CAD build for the part. Positions are in the model's coordinates, mm. A direction names the side the tool comes from. Give positions to 0.01 mm unless a question says otherwise; leave off trailing zeros. Order: outer loops, then holes, each group sorted by start corner. A loop starts at its lowest first (then second) coordinate and runs counter-clockwise, first axis right, second up. Notation, with made-up numbers: (58, 52) -> (77, 52) arc R27 cw to (77, 83) -> close; hole circle Ø5 at (20.25, -18). An arc over 180 degrees is marked (long way). Answer as CSV lines item,"result".
Autodesk Inventor part; units mm, degrees
ref_plane "YZ Plane" through (0, 0, 0) normal (1, 0, 0) x (0, 1, 0)
ref_plane "XZ Plane" through (0, 0, 0) normal (0, 1, 0) x (-1, 0, 0)
ref_plane "XY Plane" through (0, 0, 0) normal (0, 0, 1) x (1, 0, 0)
sketch "Эскиз4" plane through (0, 0, 0) normal (0, 1, 0) x (-1, 0, 0)
  line L0 (20.7, 60) -> (23.2, 6)
  line L1 (25, 6) -> (22.5, 60)
  line L2 (0, -13.2) -> (0, 79.2) construction
  line L3 (25, 6) -> (23.2, 6) construction
  line L4 (23.2, 6) -> (23.2, 0)
  line L5 (23.2, 0) -> (25, 0)
  line L6 (25, 0) -> (25, 6)
  line L7 (22.5, 60) -> (20.7, 60) construction
  line L8 (20.7, 60) -> (20.7, 66)
  line L9 (20.7, 66) -> (22.5, 66)
  line L10 (22.5, 66) -> (22.5, 60)
  line L11 (25.86, 0) -> (19.84, 0) construction
  dimension "d11" = 25
  dimension "d13" = 22.5
  dimension "d16" = 6
  dimension "d17" = 1.8
  dimension "d18" = 66
revolve "Вращение1" add sketch "Эскиз4" angle 360 about axis through (0, 0, -10) along (0, 0, 1)
properties part number "Конусный барабан катушки"
1) Wall check: line 1 along Y through (x, z) = (0, 61.9); line 2 along Y through (x, z) = (0, 2). Give the ranges that are in metal, low to high. Write a range as [from, to].
Data:
line 1,"y = [-22.5, -20.7], [20.7, 22.5]"
line 2,"y = [-25, -23.2], [23.2, 25]"
2) Band-saw the part on A-A, the plane x = 0. Write the cut outline in (y, z).
Data:
outline,"(-25, 0) -> (-23.2, 0) -> (-23.2, 6) -> (-20.7, 60) -> (-20.7, 66) -> (-22.5, 66) -> (-22.5, 60) -> (-25, 6) -> close; (20.7, 60) -> (23.2, 6) -> (23.2, 0) -> (25, 0) -> (25, 6) -> (22.5, 60) -> (22.5, 66) -> (20.7, 66) -> close"
3) Band-saw the part on D-D, the plane z = 58.5. Write the cut outline in (x, y).
Data:
outline,"circle Ø45.14 at (0, 0); hole circle Ø41.54 at (0, 0)"
4) Pull direction X, two halves, no side cores. Call faces 4 (the cylindrical face through (16.427, 12.596, 63.042)), 5 (the flat face through (-7, 20, 66)), 6 (the cylindrical face through (-23.846, -7.509, 3.042)): pulls with the +X half, pulls with the -X half, needs draft (parallel to the pull), parting line crosses it, or undercut.
Data:
face 4,"undercut"
face 5,"needs draft"
face 6,"parting line crosses it"
5) Which spindle directions (+Z, -Z, +X, -X, +Y, -Y) get a long thin tool onto all of the face, cutting with end or side? Do faces 1 (the cylindrical face through (23.178, 1.02, 2.958)), 2 (the cylindrical face through (-10.382, -19.961, 62.958)), 3 (the flat face through (-17, 17, 0)). Say none if no direction does.
Data:
face 1,"-Z"
face 2,"+Z"
face 3,"-Z, +X, -X, +Y, -Y"
6) Pin check, flat tips, straight feed: P1, Ø6, axis at x = -7, z = 9.5, coming from the -Y side; P2, Ø10, axis at y = -10.5, z = 14.5, coming from the -X side; P3, Ø4, axis at x = 2, z = 28, coming from the +Y side. Stop position of each tip, or through.
Data:
P1,"stops at y = -24.53"
P2,"stops at x = -24.01"
P3,"stops at y = 24.04"
7) Band-saw the part on C-C, the plane z = 19. Write the cut outline in (x, y).
Data:
outline,"circle Ø48.8 at (0, 0); hole circle Ø45.2 at (0, 0)"
